from build123d import *

# Parameters (mm, degrees)
F0_W     = 128.6324560642
F0_H     = 91.1146327853
F1_DEPTH = 25.4
F6_D     = 5
F3_SIZE  = 10
F5_D     = 5.5


with BuildPart() as f1:
    # F0 (on Front) → F1 (new body)
    with BuildSketch(Plane.XZ):
        Rectangle(F0_W, F0_H)
    extrude(amount=F1_DEPTH)

    # F6 (through all)
    with Locations(Plane.XZ.offset(25.4)):
        with Locations((23.9385217428, 0), (44.6983724833, -8.5433870554)):
            Hole(F6_D / 2)

    # F3
    f3_edges = [f1.edges().sort_by_distance(p)[0] for p in [
        (64.316228, -12.7, 45.557316),
        (64.316228, -12.7, -45.557316),
        (-64.316228, -12.7, -45.557316),
        (-64.316228, -12.7, 45.557316),
    ]]
    chamfer(f3_edges, length=F3_SIZE)

    # F5 (through all)
    with Locations(Plane.XZ.offset(25.4)):
        with Locations((-23.7331353128, 10.4352813214)):
            Hole(F5_D / 2)


solid = f1.part
Read the model definition and answer for the solid it produces. Units are mm, in the model's axes. Round coordinates to 2 decimals unless told otherwise and drop trailing zeros. Write each loop counter-clockwise with the first axis right and the second up, starting at its lowest first coordinate (ties: lowest second). Pieces come first, ordered by that corner, then holes.
Q1. The mould has two halves that part along X. Classify faces 1 (the face through (-59.246, -12.522, -40.627)), 2 (the face through (-25.212, -12.522, 12.754)), 3 (the face through (25.78, -12.52, 1.69)), 4 (the face through (59.386, -12.522, -40.487)): released by +X, released by -X, zero draft, split by the parting line, or undercut.
Values:
face 1: released by -X
face 2: undercut
face 3: undercut
face 4: released by +X
Q2. Find section B-B on x = 45. Determine the outline of the cut face in (y, z), and give its area (3 significant figures).
Values:
outline: (-25.4, -45.56) - (0, -45.56) - (0, -11.03) - (-25.4, -11.03) - close; (-25.4, -6.06) - (0, -6.06) - (0, 45.56) - (-25.4, 45.56) - close
area: 2,190 mm2
Q3. Find section C-C on y = -16.25. Determine the outline of the cut face in (x, z).
Values:
outline: (-64.32, -35.56) - (-54.32, -45.56) - (54.32, -45.56) - (64.32, -35.56) - (64.32, 35.56) - (54.32, 45.56) - (-54.32, 45.56) - (-64.32, 35.56) - close; hole circle Ø5.5 at (-23.73, 10.44); hole circle Ø5 at (23.94, 0); hole circle Ø5 at (44.7, -8.54)
Q4. Straight lines are drawn through the part: line 1 (X direction, y = -19.25, z = 11.5); line 2 (X direction, y = -15.5, z = -7.5); line 3 (X direction, y = -5, z = -36). For each, find the intervals that lie inside material, in ascending order.
Values:
line 1: x = -64.32 to -26.27, -21.2 to 64.32
line 2: x = -64.32 to 42.43, 46.97 to 64.32
line 3: x = -63.87 to 63.87
Q5. Find section A-A on z = 0. Determine the outline of the cut face in (x, y).
Values:
outline: (-64.32, -25.4) - (21.44, -25.4) - (21.44, 0) - (-64.32, 0) - close; (26.44, -25.4) - (64.32, -25.4) - (64.32, 0) - (26.44, 0) - close
